Drawing for the job (mm, zero at the part's lowest x, y, z). A direction names the side the tool comes from. Give positions to 0.01 mm unless a question says otherwise; leave off trailing zeros. Order: outer loops, then holes, each group sorted by start corner. A loop starts at its lowest first (then second) coordinate and runs counter-clockwise, first axis right, second up. Notation, with made-up numbers: M 88.25,-4 L 125.25,-4 A30 ccw 125.25,27 Z; hole C -25,-36.75 d1. An arc over 180 degrees is marked long. Answer as a JSON object with one key per item and string values.
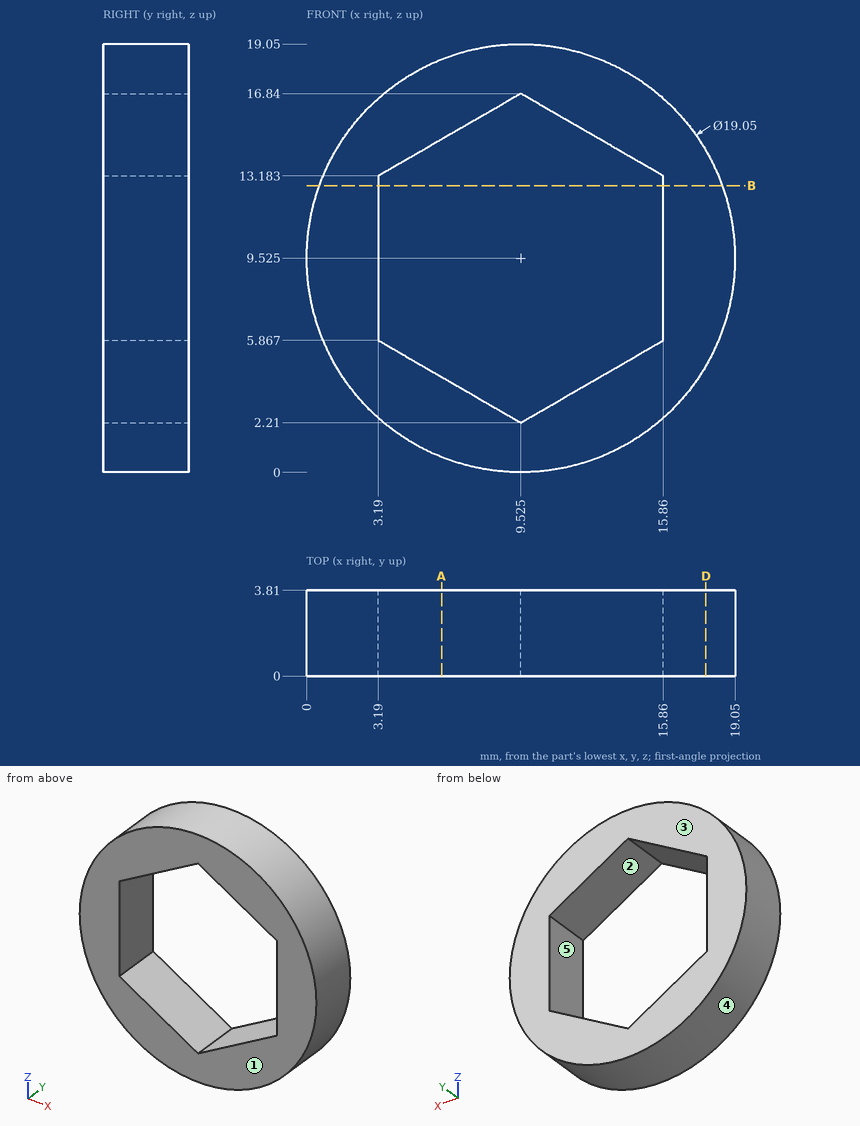
1. Pin check, flat tip, straight feed: P1, Ø1, axis at y = 0.5, z = 4, coming from the -X side. Stop position of the tip, or through.
Worked answers:
{"P1": "stops at x = 1.43"}
2. Cut at B-B on z = 12.75. Give the cut face in (x, y).
Worked answers:
{"outline": "M 0.56,0 L 3.19,0 L 3.19,3.81 L 0.56,3.81 Z; M 15.86,0 L 18.49,0 L 18.49,3.81 L 15.86,3.81 Z"}
3. Cut at A-A on x = 6. Give the cut face in (y, z) (1 decimal).
Worked answers:
{"outline": "M 0,0.7 L 3.8,0.7 L 3.8,4.2 L 0,4.2 Z; M 0,14.8 L 3.8,14.8 L 3.8,18.4 L 0,18.4 Z"}
4. Which spindle directions (+Z, -Z, +X, -X, +Y, -Y) get a long thin tool onto all of the face, cutting with end or side? Do the marked faces 1 and 2. Say none if no direction does.
Worked answers:
{"face 1": "+Z, -Z, +X, -X, -Y", "face 2": "+Y, -Y"}
5. Two-plate mould, pull along Z, no slides. Class the marked faces 3, 4 and 5: +Z half, -Z half, draft (parallel to the pull), parting line (faces both ways), or undercut.
Worked answers:
{"face 3": "draft", "face 4": "parting line", "face 5": "undercut"}
6. Cut at D-D on x = 17.75. Give the cut face in (y, z), plus the area to 3 significant figures.
Worked answers:
{"outline": "M 0,4.72 L 3.81,4.72 L 3.81,14.33 L 0,14.33 Z", "area": "36.6 mm^2"}
7. Probe line 1 along Z through (x, y) = (13.75, 0.9); line 2 along Z through (x, y) = (9.25, 3.3) (1 decimal); line 3 along X through (y, z) = (2.6, 15.75) (1 decimal). List the from-to ranges inside material, lowest first.
Worked answers:
{"line 1": "z = 0.99 to 4.65, 14.4 to 18.06", "line 2": "z = 0 to 2.4, 16.7 to 19", "line 3": "x = 2.3 to 7.6, 11.4 to 16.7"}
